```python
from build123d import *

# Parameters (mm, degrees)
ESQUISSE1_W             = 35
ESQUISSE1_H             = 31
BOSS_EXTRU_1_DEPTH      = 16
ENL_V_MAT_EXTRU_1_DEPTH = 35
ESQUISSE3_R             = 1.75
ENL_V_MAT_EXTRU_2_DEPTH = 5
ESQUISSE4_R             = 2.75
ENL_V_MAT_EXTRU_3_DEPTH = 3


with BuildPart() as part:
    # Esquisse1 → Boss.-Extru.1 (new body)
    with BuildSketch(Plane.XY):
        Rectangle(ESQUISSE1_W, ESQUISSE1_H)
    extrude(amount=BOSS_EXTRU_1_DEPTH)

    # Esquisse2 → Enlèv. mat.-Extru.1 (cut)
    with BuildSketch(Plane.ZY.offset(17.5)):
        Polygon((5, 13.5), (5, -13.5), (14, -13.5), (14, -4.5), (16, -4.5), (16, 4.5), (14, 4.5), (14, 13.5), align=None)
    extrude(amount=-ENL_V_MAT_EXTRU_1_DEPTH, mode=Mode.SUBTRACT)

    # Esquisse3 → Enlèv. mat.-Extru.2 (cut)
    with BuildSketch(Plane.XY.offset(5)):
        Circle(ESQUISSE3_R)
    extrude(amount=-ENL_V_MAT_EXTRU_2_DEPTH, mode=Mode.SUBTRACT)

    # Esquisse4 → Enlèv. mat.-Extru.3 (cut)
    with BuildSketch(Plane.XY.offset(5)):
        Circle(ESQUISSE4_R)
    extrude(amount=-ENL_V_MAT_EXTRU_3_DEPTH, mode=Mode.SUBTRACT)


solid = part.part
```
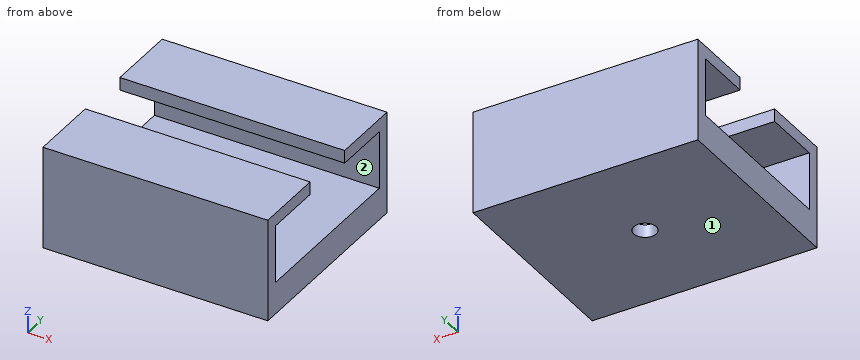
The listing builds one solid part. Answer for the finished solid, in the listing's coordinates (mm). Face numbers are marked on the shaded views. A direction names the side the tool comes from. Give positions to 0.01 mm unless a question says otherwise; leave off trailing zeros. Order: outer loops, then holes, each group sorted by start corner. A loop starts at its lowest first (then second) coordinate and runs counter-clockwise, first axis right, second up. Notation, with made-up numbers: (78, 75.5) -> (112, 75.5) arc R24 ccw to (112, 114.5) -> close; hole circle Ø6 at (9.25, 46.25). An arc over 180 degrees is marked (long way). Answer as a JSON object with one key per item and string values. Group by question number.
Item 1: The part is cut by section C-C on x = 0. Write down the section's boundary in (y, z), and give its area (4 significant figures).
Item 2: Consider L1, parallel to Z at x = -7.5, y = -5; L2, parallel to Y at x = -11, z = 9.5; L3, parallel to Y at x = 0, z = 4.2. Determine where each line is inside the solid, lowest interval first. Write a range as from..to.
Item 3: Flat-ended cylindrical pins translate along their axes: pin 1 (4.5 mm diameter, centred on x = 0, y = 0, fed in from +Z); pin 2 (5 mm diameter, centred on y = 1.5, z = 13, fed in from +X); pin 3 (4.5 mm diameter, centred on x = -0.5, y = 0.5, fed in from +Z). Find the tip coordinate at first contact, or state that the pin passes through.
Item 4: The part is cut by section B-B on y = -5.5. Write down the section's boundary in (x, z).
Item 5: The part is cut by section A-A on z = 8.5. Write down the section's boundary in (x, y), and give its area (3 significant figures).
Item 6: The part is cut by section D-D on x = 13. Write down the section's boundary in (y, z).
Item 7: A tool of negligible diameter and unlimited length cuts with its end or side. For the marked faces 1 and 2, from which of +Z, -Z, +X, -X, +Y, -Y can it reach the whole face along a straight path? Write none if from no direction.
Result set:
{
 "1": {"outline": "(-15.5, 0) -> (-1.75, 0) -> (-1.75, 2) -> (-2.75, 2) -> (-2.75, 5) -> (-13.5, 5) -> (-13.5, 14) -> (-4.5, 14) -> (-4.5, 16) -> (-15.5, 16) -> close; (1.75, 0) -> (15.5, 0) -> (15.5, 16) -> (4.5, 16) -> (4.5, 14) -> (13.5, 14) -> (13.5, 5) -> (2.75, 5) -> (2.75, 2) -> (1.75, 2) -> close", "area": "211.5 mm²"},
 "2": {"L1": "0..5, 14..16", "L2": "-15.5..-13.5, 13.5..15.5", "L3": "-15.5..-2.75, 2.75..15.5"},
 "3": {"pin 1": "z = 2", "pin 2": "through", "pin 3": "z = 5"},
 "4": {"outline": "(-17.5, 0) -> (17.5, 0) -> (17.5, 5) -> (-17.5, 5) -> close; (-17.5, 14) -> (17.5, 14) -> (17.5, 16) -> (-17.5, 16) -> close"},
 "5": {"outline": "(-17.5, -15.5) -> (17.5, -15.5) -> (17.5, -13.5) -> (-17.5, -13.5) -> close; (-17.5, 13.5) -> (17.5, 13.5) -> (17.5, 15.5) -> (-17.5, 15.5) -> close", "area": "140 mm²"},
 "6": {"outline": "(-15.5, 0) -> (15.5, 0) -> (15.5, 16) -> (4.5, 16) -> (4.5, 14) -> (13.5, 14) -> (13.5, 5) -> (-13.5, 5) -> (-13.5, 14) -> (-4.5, 14) -> (-4.5, 16) -> (-15.5, 16) -> close"},
 "7": {"face 1": "-Z, +X, -X, +Y, -Y", "face 2": "+X, -X"}
}
